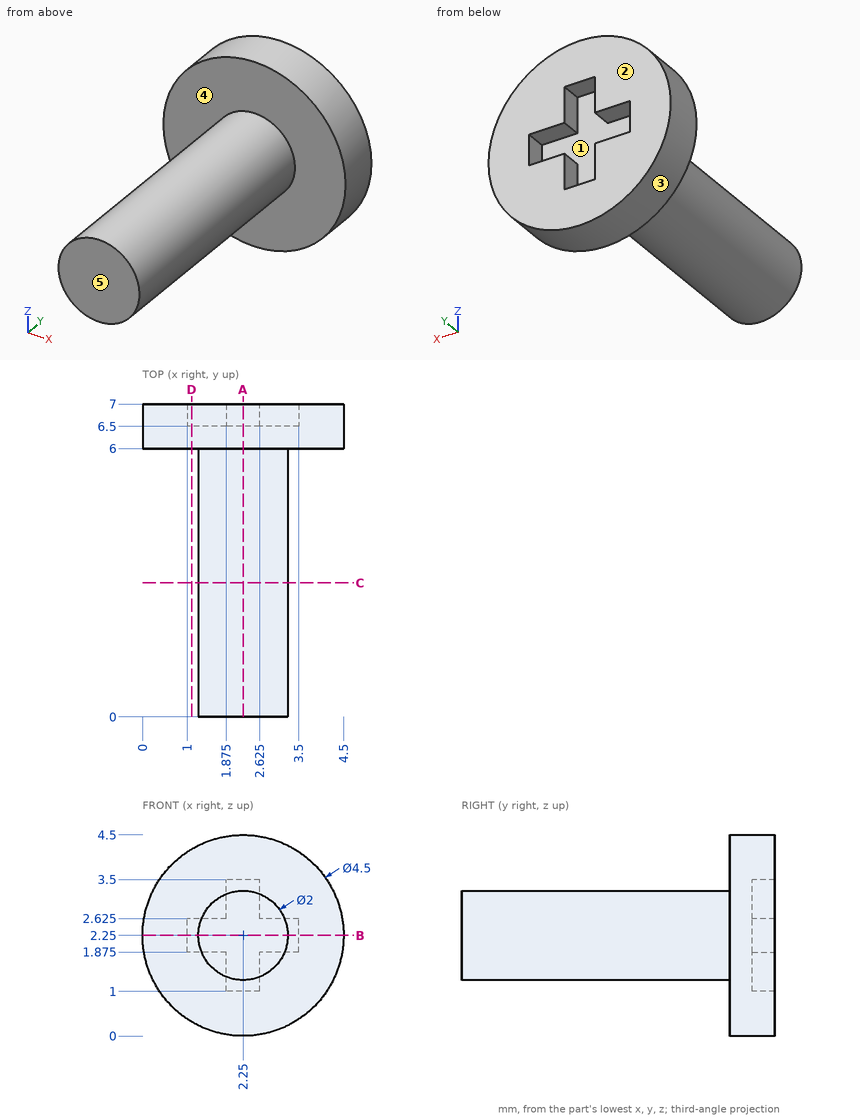
Answer from the drawing. Dimensions are ordinates in mm from the lowest x, y and z of the part. A direction names the side the tool comes from. Give positions to 0.01 mm unless a question says otherwise; leave off trailing zeros. Write each loop counter-clockwise with the first axis right and the second up, starting at its lowest first coordinate (ties: lowest second). Pieces come first, ordered by that corner, then holes. Notation, with made-up numbers: M 16,66.25 L 48,66.25 A7 ccw 48,78.25 Z; hole C 50,12.25 d1. An arc over 180 degrees is marked long. Answer as CSV lines item,"result".
Q1. A cutting plane is placed at A-A on x = 2.25. Write down the section's boundary in (y, z).
A:
outline,"M 0,1.25 L 6,1.25 L 6,0 L 7,0 L 7,1 L 6.5,1 L 6.5,3.5 L 7,3.5 L 7,4.5 L 6,4.5 L 6,3.25 L 0,3.25 Z"
Q2. A cutting plane is placed at C-C on y = 3. Write down the section's boundary in (x, z), plus the area to 3 significant figures.
A:
outline,"C 2.25,2.25 d2"
area,"3.14 mm²"
Q3. The mould has two halves that part along X. Classify the marked faces 1, 2 and 3: +X half, -X half, draft (parallel to the pull), parting line (faces both ways), or undercut.
A:
face 1,"undercut"
face 2,"draft"
face 3,"parting line"
Q4. A cutting plane is placed at B-B on z = 2.25. Write down the section's boundary in (x, y), plus the area to 4 significant figures.
A:
outline,"M 0,6 L 1.25,6 L 1.25,0 L 3.25,0 L 3.25,6 L 4.5,6 L 4.5,7 L 3.5,7 L 3.5,6.5 L 1,6.5 L 1,7 L 0,7 Z"
area,"15.25 mm²"
Q5. A tool of negligible diameter and unlimited length cuts with its end or side. For the marked faces 4 and 5, from which of +Z, -Z, +X, -X, +Y, -Y can it reach the whole face along a straight path? Write none if from no direction.
A:
face 4,"-Y"
face 5,"+Z, -Z, +X, -X, -Y"
Q6. A cutting plane is placed at D-D on x = 1.1. Write down the section's boundary in (y, z) (3 decimals).
A:
outline,"M 6,0.316 L 7,0.316 L 7,1.875 L 6.5,1.875 L 6.5,2.625 L 7,2.625 L 7,4.184 L 6,4.184 Z"
Q7. Find the intervals of material crossed by probe 1 along Y at (x, z) = (0.95, 0.6); probe 2 along Y at (x, z) = (2.95, 2.2); probe 3 along X at (y, z) = (6.75, 1.95), in increasing order. Write a range as [from, to].
A:
probe 1,"y = [6, 7]"
probe 2,"y = [0, 6.5]"
probe 3,"x = [0.02, 1], [3.5, 4.48]"
Q8. Given P1, Ø2, axis at x = 3, y = 2, coming from the -Z side; P2, Ø0.6, axis at x = 1.5, y = 7, coming from the -Z side; P3, Ø1.5, axis at x = 0.5, z = 3, coming from the -Y side, each flat-ended and moving along its own axis, determine where each tip first touches the part or whether it passes through.
A:
P1,"stops at z = 1.25"
P2,"stops at z = 0.05"
P3,"stops at y = 6"
